```python
from build123d import *

# Parameters (mm, degrees)
PAD_DEPTH       = 110
SKETCH001_R     = 2.5
POCKET_DEPTH    = 5
SKETCH002_R     = 50
POCKET001_DEPTH = 2
FILLET_R        = 5
FILLET001_R     = 1
FILLET002_R     = 1
FILLET003_R     = 1
FILLET004_R     = 1


with BuildPart() as part:
    # Sketch → Pad (new body)
    with BuildSketch(Plane.XY):
        Polygon((0, 40), (0, 0), (120, 0), (120, 20), (115, 20), (115, 5), (5, 5), (5, 40), align=None)
    extrude(amount=PAD_DEPTH)

    # Sketch001 (on Face1 of Pad) → Pocket (cut)
    with BuildSketch(Plane(origin=(0, 0, 0), x_dir=(0, -1, 0), z_dir=(-1, 0, 0))):
        with Locations((-20, 80)):
            Circle(SKETCH001_R)
        with Locations((-20, 30)):
            Circle(SKETCH001_R)
    extrude(amount=-POCKET_DEPTH, mode=Mode.SUBTRACT)

    # Sketch002 (on Face12 of Pocket) → Pocket001 (cut)
    with BuildSketch(Plane(origin=(0, 5, 0), x_dir=(-1, 0, 0), z_dir=(0, 1, 0))):
        with Locations((-60, 55)):
            Circle(SKETCH002_R)
    extrude(amount=-POCKET001_DEPTH, mode=Mode.SUBTRACT)

    # Fillet
    fillet_edges = [part.edges().sort_by_distance(p)[0] for p in [
        (120, 0, 55),
    ]]
    fillet(fillet_edges, radius=FILLET_R)

    # Fillet001
    fillet001_edges = [part.edges().sort_by_distance(p)[0] for p in [
        (57.5, 0, 110),
    ]]
    fillet(fillet001_edges, radius=FILLET001_R)

    # Fillet002
    fillet002_edges = [part.edges().sort_by_distance(p)[0] for p in [
        (57.5, 0, 0),
    ]]
    fillet(fillet002_edges, radius=FILLET002_R)

    # Fillet003
    fillet003_edges = [part.edges().sort_by_distance(p)[0] for p in [
        (120, 20, 55),
    ]]
    fillet(fillet003_edges, radius=FILLET003_R)

    # Fillet004
    fillet004_edges = [part.edges().sort_by_distance(p)[0] for p in [
        (115, 20, 55),
        (5, 40, 55),
        (60, 5, 110),
        (5, 22.5, 110),
        (115, 12, 110),
        (115, 12, 0),
        (60, 5, 0),
        (5, 22.5, 0),
        (2.5, 40, 0),
        (2.5, 40, 110),
    ]]
    fillet(fillet004_edges, radius=FILLET004_R)


solid = part.part
```
Could you check a few things on this model? Use its own coordinates, in mm. A direction names the side the tool comes from. Give positions to 0.01 mm unless a question says otherwise; leave off trailing zeros. Loops run counter-clockwise (first coordinate to the right, second up) from the corner with the lowest first, then second, coordinate; pieces in that order, holes last. Notation, with made-up numbers: (72, 29) - (90, 29) arc R15 cw to (90, 53) - close; hole circle Ø11 at (71, 42.25). An arc over 180 degrees is marked (long way). Answer in a Markdown table with one row per item. Add a question column.
Q1. If we section it at B-B (z = 55): List the corners of the cut face in (x, y) for me.
Q2. For pin 1 (1.5 mm diameter, centred on x = 118, z = 49.5, fed in from +Y); pin 2 (5 mm diameter, centred on x = 39, z = 27.5, fed in from +Y); pin 3 (4 mm diameter, centred on y = 20, z = 30, fed in from -X); pin 4 (8 mm diameter, centred on x = 53.5, y = 12.5, fed in from +Z), each with a flat end and sliding along its axis, tell me the tip position at first contact or that it passes through.
Q3. We'd pull the mould along Z, two halves only. Please class faces 1 (the face through (115, 12, 54)), 2 (the face through (50, 3, 0)), 3 (the face through (2.46, 21.84, 31.69)): +Z half, -Z half, draft (parallel to the pull), parting line (faces both ways), or undercut.
Q4. Which directions (+Z, -Z, +X, -X, +Y, -Y) give clear straight access to the entire face, cutting with the end or side of a thin tool? Please do faces 4 (the face through (2.5, 22.5, 80.1)), 5 (the face through (85, 5, 99)), 6 (the face through (61, 3, 56)), 7 (the face through (118, 20, 54)).
Q5. If we section it at D-D (z = 30): List the corners of the cut face in (x, y) for me, plus the area to 3 significant figures.
Q6. If we section it at C-C (x = 20): List the corners of the cut face in (y, z) for me.
Q7. Please list where these lines run through material, in increasing order: L1, parallel to Z at x = 3.1, y = 20; L2, parallel to X at y = 7, z = 87.5; L3, parallel to Z at x = 60, y = 3.75. Write a range as from..to.
Q8. If we section it at A-A (y = 10): List the corners of the cut face in (x, z) for me.
The answers:
| question | item | result |
|---|---|---|
| 1 | outline | (0, 0) - (115, 0) arc R5 ccw to (120, 5) - (120, 19) arc R1 ccw to (119, 20) - (116, 20) arc R1 ccw to (115, 19) - (115, 5) - (110, 5) - (110, 3) - (10, 3) - (10, 5) - (5, 5) - (5, 39) arc R1 ccw to (4, 40) - (0, 40) - close |
| 2 | pin 1 | stops at y = 20 |
| 2 | pin 2 | stops at y = 3 |
| 2 | pin 3 | stops at x = 115 |
| 2 | pin 4 | passes through |
| 3 | face 1 | draft |
| 3 | face 2 | -Z half |
| 3 | face 3 | undercut |
| 4 | face 4 | -X |
| 4 | face 5 | +Z, -Z, +Y |
| 4 | face 6 | +Y |
| 4 | face 7 | +Z, -Z, +X, +Y |
| 5 | outline | (0, 0) - (115, 0) arc R5 ccw to (120, 5) - (120, 19) arc R1 ccw to (119, 20) - (116, 20) arc R1 ccw to (115, 19) - (115, 5) - (103.3, 5) - (103.3, 3) - (16.7, 3) - (16.7, 5) - (5, 5) - (5, 17.5) - (0, 17.5) - close; (0, 22.5) - (5, 22.5) - (5, 39) arc R1 ccw to (4, 40) - (0, 40) - close |
| 5 | area | 646 mm^2 |
| 6 | outline | (0, 1) arc R1 ccw to (1, 0) - (4, 0) arc R1 ccw to (5, 1) - (5, 25) - (3, 25) - (3, 85) - (5, 85) - (5, 109) arc R1 ccw to (4, 110) - (1, 110) arc R1 ccw to (0, 109) - close |
| 7 | L1 | z = 0..27.5, 32.5..77.5, 82.5..110 |
| 7 | L2 | x = 0..5, 115..120 |
| 7 | L3 | z = 0..5, 105..110 |
| 8 | outline | (0, 0) - (4, 0) arc R1 ccw to (5, 1) - (5, 109) arc R1 ccw to (4, 110) - (0, 110) - close; (115, 1) arc R1 ccw to (116, 0) - (119, 0) arc R1 ccw to (120, 1) - (120, 109) arc R1 ccw to (119, 110) - (116, 110) arc R1 ccw to (115, 109) - close |
